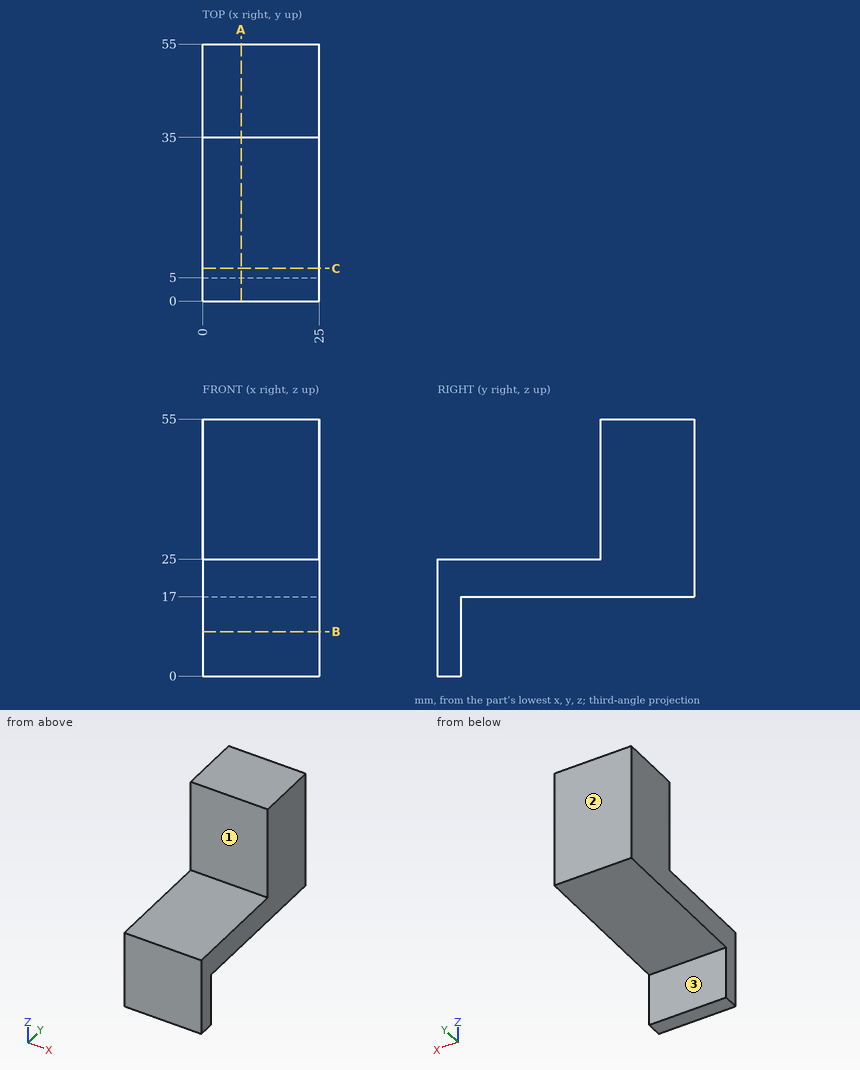
Answer from the drawing. Dimensions are ordinates in mm from the lowest x, y and z of the part. A direction names the side the tool comes from. Coordinates: 2 decimals unless noted, no trailing zeros. Loops run counter-clockwise (first coordinate to the right, second up) from the corner with the lowest first, then second, coordinate; pieces in that order, holes last. Notation, with made-up numbers: (40, -13) -> (50, -13) arc R5 cw to (50, -6) -> close; hole circle Ø7 at (-29.75, 13.25). An arc over 180 degrees is marked (long way). Answer in a Markdown table with one row per item.
Item 1: For the marked faces 1, 2 and 3, determine the directions among +Z, -Z, +X, -X, +Y, -Y from which every point of the face is accessible in a straight line to the end or side of a thin tool.
Returned:
| item | result |
|---|---|
| face 1 | +Z, +X, -X, -Y |
| face 2 | +Z, -Z, +X, -X, +Y |
| face 3 | -Z, +X, -X, +Y |
Item 2: A cutting plane is placed at B-B on z = 9.5. Determine the outline of the cut face in (x, y), plus the area to 3 significant figures.
Returned:
| item | result |
|---|---|
| outline | (0, 0) -> (25, 0) -> (25, 5) -> (0, 5) -> close |
| area | 125 mm^2 |
Item 3: Straight lines are drawn through the part: line 1 along Y through (x, z) = (13.25, 30.5); line 2 along Z through (x, y) = (14.5, 31); line 3 along Z through (x, y) = (8.5, 41.5). For each, find the intervals that lie inside material, in ascending order. Write a range as [from, to].
Returned:
| item | result |
|---|---|
| line 1 | y = [35, 55] |
| line 2 | z = [17, 25] |
| line 3 | z = [17, 55] |
Item 4: Each of these flat-tipped pins is pushed along its axis until it touches: P1, Ø1.5, axis at x = 14, z = 28.5, coming from the -Y side; P2, Ø12.5, axis at x = 11, y = 25.5, coming from the -Z side; P3, Ø3, axis at x = 21.5, y = 20.5, coming from the +Z side. Where does it stop, or does it pass through?
Returned:
| item | result |
|---|---|
| P1 | stops at y = 35 |
| P2 | stops at z = 17 |
| P3 | stops at z = 25 |
Item 5: A cutting plane is placed at C-C on y = 7. Determine the outline of the cut face in (x, z).
Returned:
| item | result |
|---|---|
| outline | (0, 17) -> (25, 17) -> (25, 25) -> (0, 25) -> close |
Item 6: A cutting plane is placed at A-A on x = 8.25. Determine the outline of the cut face in (y, z), plus the area to 4 significant figures.
Returned:
| item | result |
|---|---|
| outline | (0, 0) -> (5, 0) -> (5, 17) -> (55, 17) -> (55, 55) -> (35, 55) -> (35, 25) -> (0, 25) -> close |
| area | 1,125 mm^2 |
